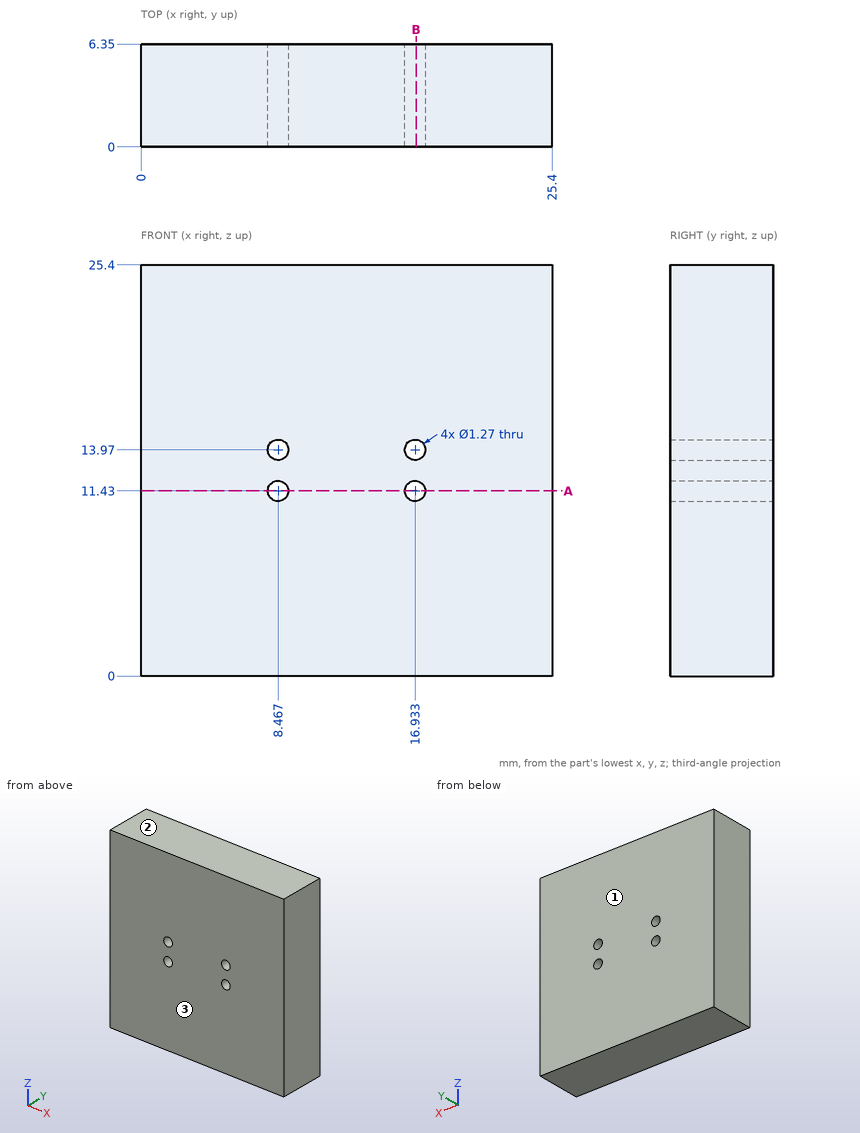
For this review, use the dimensioned drawing (mm, ordinates from the lowest corner) and the shaded views. Round coordinates to 2 decimals unless told otherwise and drop trailing zeros. Write each loop counter-clockwise with the first axis right and the second up, starting at its lowest first coordinate (ties: lowest second). Pieces come first, ordered by that corner, then holes. Notation, with made-up numbers: (0, 29.5) - (25, 29.5) arc R19 ccw to (25, 58.5) - close; hole circle Ø11 at (-24.5, -2.5). An arc over 180 degrees is marked (long way). One line per item, written item: value. Start each with the question number.
1. Consider section A-A on z = 11.43. Write out the cut boundary in (x, y), and give its area (3 significant figures).
2. To check wall thickness, follow L1, parallel to X at y = 3.25, z = 11.43; L2, parallel to X at y = 1, z = 13.5 (1 decimal); L3, parallel to Z at x = 17.5, y = 1 (1 decimal). State the ranges of each line that lie inside material, in increasing order. Write a range as from..to.
3. The part is to be moulded in two halves that separate along Y. For the marked faces 1, 2 and 3, say which applies: released by +Y, released by -Y, zero draft, split by the parting line, or undercut.
4. Consider section B-B on x = 17. Write out the cut boundary in (y, z), and give its area (3 significant figures).
Checks:
1. outline: (0, 0) - (7.83, 0) - (7.83, 6.35) - (0, 6.35) - close; (9.1, 0) - (16.3, 0) - (16.3, 6.35) - (9.1, 6.35) - close; (17.57, 0) - (25.4, 0) - (25.4, 6.35) - (17.57, 6.35) - close
1. area: 145 mm^2
2. L1: x = 0..7.83, 9.1..16.3, 17.57..25.4
2. L2: x = 0..8, 8.9..16.5, 17.4..25.4
2. L3: z = 0..11.1, 11.7..13.7, 14.3..25.4
3. face 1: released by +Y
3. face 2: zero draft
3. face 3: released by -Y
4. outline: (0, 0) - (6.35, 0) - (6.35, 10.8) - (0, 10.8) - close; (0, 12.06) - (6.35, 12.06) - (6.35, 13.34) - (0, 13.34) - close; (0, 14.6) - (6.35, 14.6) - (6.35, 25.4) - (0, 25.4) - close
4. area: 145 mm^2
